Could you check a few things on this drawing? It's one solid part, dimensions in mm from its lowest x, y, z. Coordinates: 2 decimals unless noted, no trailing zeros. Loops run counter-clockwise (first coordinate to the right, second up) from the corner with the lowest first, then second, coordinate; pieces in that order, holes last. Notation, with made-up numbers: M -30,32.5 L -5,32.5 A22 cw -5,67.5 Z; hole C 51.25,37 d8. An arc over 180 degrees is marked long. Answer as a JSON object with one key per item and string values. Group by question number.
Item 1: If I drill on line 1 (Y direction, x = 5, z = 1.35); line 2 (X direction, y = 65, z = 3.85); line 3 (Z direction, x = 57.5, y = 64), over which ranges is the centre line in solid material (lowest first)?
Item 2: Suppose I cut it at A-A (y = 24). Write out the boundary of the cut face in (x, z), then the cut area to 3 significant figures.
Item 3: Suppose I cut it at B-B (x = 117). Write out the boundary of the cut face in (y, z).
Item 4: I'm going to push flat-ended pins straight in: pin 1 Ø1.5 at (x, z) = (85, 7) entering from +Y; pin 2 Ø0.9 at (x, z) = (144.5, 6.5) entering from -Y; pin 3 Ø3.5 at (x, y) = (5, 5) entering from +Z. Where does each tip first touch, or does it pass through?
Item 5: Suppose I cut it at C-C (z = 6.5). Write out the boundary of the cut face in (x, y).
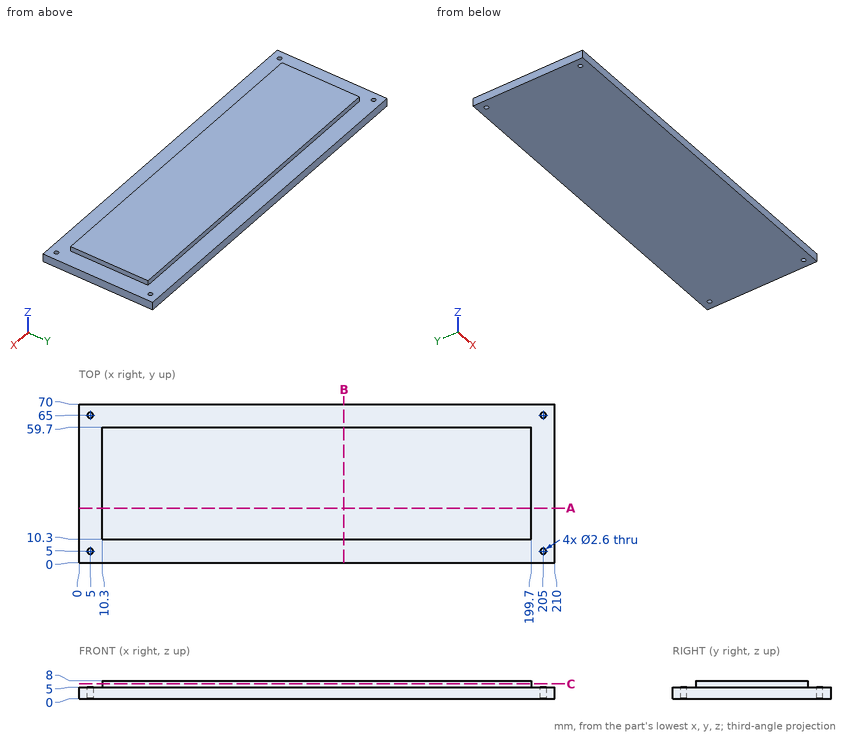
From the geometry:
{
 "1": {"line 1": "0 to 3.7, 6.3 to 63.7, 66.3 to 70", "line 2": "0 to 3.7, 6.3 to 203.7, 206.3 to 210", "line 3": "0 to 5"},
 "2": {"outline": "M 0,0 L 210,0 L 210,5 L 199.7,5 L 199.7,8 L 10.3,8 L 10.3,5 L 0,5 Z", "area": "1,620 mm2"},
 "3": {"outline": "M 0,0 L 70,0 L 70,5 L 59.7,5 L 59.7,8 L 10.3,8 L 10.3,5 L 0,5 Z"},
 "4": {"pin 1": "y = 59.7", "pin 2": "y = 10.3", "pin 3": "z = 5"},
 "5": {"outline": "M 10.3,10.3 L 199.7,10.3 L 199.7,59.7 L 10.3,59.7 Z"}
}
